Read the model definition and answer for the solid it produces. Units are mm, in the model's axes. A direction names the side the tool comes from. Coordinates: 2 decimals unless noted, no trailing zeros. Loops run counter-clockwise (first coordinate to the right, second up) from the corner with the lowest first, then second, coordinate; pieces in that order, holes last. Notation, with made-up numbers: M 58.25,58 L 80.25,58 A13 ccw 80.25,72 Z; hole C -32.5,-12 d4. An arc over 180 degrees is marked long. Put each result on its own line as item: value.
from build123d import *

# Parameters (mm, degrees)
F0_W     = 18
F0_H     = 3.5
F1_DEPTH = 10
F2_W     = 8
F2_H     = 6
F3_DEPTH = 25
F4_DEPTH = 21.2
F6_DEPTH = 18
F7_R     = 1
F8_DEPTH = 25


with BuildPart() as f1:
    # F0 (on Front) → F1 (new body)
    with BuildSketch(Plane.XZ):
        Rectangle(F0_W, F0_H)
    extrude(amount=F1_DEPTH)

    # F2 (on Top) → F3 (cut)
    with BuildSketch(Plane.XY):
        Rectangle(F2_W, F2_H)
    extrude(amount=-F3_DEPTH, mode=Mode.SUBTRACT)

    # F2 (on Top) → F4 (cut)
    with BuildSketch(Plane.XY):
        Rectangle(F2_W, F2_H)
    extrude(amount=F4_DEPTH, mode=Mode.SUBTRACT)

    # F5 (on face) → F6 (intersect)
    with BuildSketch(Plane.YZ.offset(9)):
        with BuildLine():
            ThreePointArc((0, 1.55), (-2.498001, 1.69998), (-5, 1.75))
            Line((-5, 1.75), (-5, -1.55))
            ThreePointArc((-5, -1.55), (-2.498001, -1.60002), (0, -1.75))
            Line((0, -1.75), (0, 1.55))
        make_face()
        with BuildLine():
            Line((-5, -1.55), (-5, 1.75))
            ThreePointArc((-5, 1.75), (-7.501999, 1.69998), (-10, 1.55))
            Line((-10, 1.55), (-10, -1.75))
            ThreePointArc((-10, -1.75), (-7.501999, -1.60002), (-5, -1.55))
        make_face()
    extrude(amount=-F6_DEPTH, mode=Mode.INTERSECT)

    # F7 (on face) → F8 (cut)
    with BuildSketch(Plane(origin=(-9, 0, 0), x_dir=(0, -1, 0), z_dir=(-1, 0, 0))):
        with BuildLine():
            ThreePointArc((1, -0.75), (1.5, -1.25), (2, -0.75))
            ThreePointArc((2, -0.75), (1.5, -0.25), (1, -0.75))
        make_face()
        with Locations((8.5, -0.25)):
            Circle(F7_R)
    extrude(amount=-F8_DEPTH, mode=Mode.SUBTRACT)


solid = f1.part
1) Find section A-A, the plane x = 7.25. Write down the section's boundary in (y, z), plus the area to 3 significant figures.
Answer list:
outline: M -10,-1.75 A62.6 cw -5,-1.55 A62.6 cw 0,-1.75 L 0,1.55 A62.6 ccw -5,1.75 A62.6 ccw -10,1.55 Z; hole C -8.5,-0.25 d2; hole C -1.5,-0.75 d1
area: 29.1 mm^2
2) Determine the mould class of faces 3 (the cylindrical face through (-6.54, -1.1, -1.05)), 4 (the cylindrical face through (6.46, -1.1, -1.05)), 5 (the flat face through (4, -2, 0)) for opening direction Z: released by +Z, released by -Z, zero draft, split by the parting line, or undercut.
Answer list:
face 3: undercut
face 4: undercut
face 5: zero draft
3) Straight lines are drawn through the part: line 1 (X direction, y = -2.25, z = -1); line 2 (Y direction, x = 7.5, z = -0.8); line 3 (Z direction, x = 6.5, y = -5). For each, find the intervals that lie inside material, in ascending order. Write a range as [from, to].
Answer list:
line 1: x = [-9, -4], [4, 9]
line 2: y = [-10, -9.34], [-7.66, -2], [-1, 0]
line 3: z = [-1.55, 1.75]
4) Find section B-B, the plane z = 1. Write down the section's boundary in (x, y), plus the area to 3 significant figures.
Answer list:
outline: M -9,-10 L 9,-10 L 9,0 L 4,0 L 4,-3 L -4,-3 L -4,0 L -9,0 Z
area: 156 mm^2
5) Which of the six approach directions +Z, -Z, +X, -X, +Y, -Y give full straight-line access (tool end or side, diameter ignored) to faces 1 (the flat face through (0, -10, 0)), 2 (the flat face through (0, -3, 0))?
Answer list:
face 1: +Z, -Z, +X, -X, -Y
face 2: +Z, -Z, +Y
6) Find section C-C, the plane y = -8.75. Write down the section's boundary in (x, z), plus the area to 3 significant figures.
Answer list:
outline: M -9,-1.66 L 9,-1.66 L 9,-1.22 L -9,-1.22 Z; M -9,0.72 L 9,0.72 L 9,1.64 L -9,1.64 Z
area: 24.5 mm^2
7) Find section D-D, the plane x = -1.5. Write down the section's boundary in (y, z), plus the area to 3 significant figures.
Answer list:
outline: M -10,-1.75 A62.6 cw -5,-1.55 A62.6 cw -3,-1.58 L -3,1.72 A62.6 ccw -5,1.75 A62.6 ccw -10,1.55 Z; hole C -8.5,-0.25 d2
area: 20.0 mm^2
8) Given pin 1 Ø1 at (x, y) = (-3, -3.5) entering from -Z; pin 2 Ø1.6 at (x, z) = (0.5, -0.5) entering from +Y; pin 3 Ø1.8 at (y, z) = (-8.5, -0.25) entering from -X, each flat-ended and moving along its own axis, determine where each tip first touches the part or whether it passes through.
Answer list:
pin 1: stops at z = -1.58
pin 2: stops at y = -3
pin 3: passes through
